from build123d import *

# Parameters (mm, degrees)
SKETCH_1_W             = 30
SKETCH_1_H             = 250
EXTRUDE_1_DEPTH        = 3
EXTRUDE_2_DEPTH        = 15
PATTERN_LINEAR_1_COUNT = 35
PATTERN_LINEAR_1_PITCH = 7


with BuildPart() as part:
    # 스케치1 → 보스-돌출1 (new body)
    with BuildSketch(Plane(origin=(0, 0, 0), x_dir=(1, 0, 0), z_dir=(0, 1, 0))):
        Rectangle(SKETCH_1_W, SKETCH_1_H)
    extrude(amount=EXTRUDE_1_DEPTH)

    # 스케치3 → 보스-돌출2 (add, symmetric)
    with BuildSketch(Plane(origin=(0, 0, 0), x_dir=(0, 0, -1), z_dir=(1, 0, 0))):
        Polygon((-125, 3), (-118, 6), (-118, 3), align=None)
    extrude_2 = extrude(amount=EXTRUDE_2_DEPTH, both=True)

    # 선형 패턴1: 보스-돌출2 ×35
    with Locations(*[(0, 0, -i * PATTERN_LINEAR_1_PITCH) for i in range(1, PATTERN_LINEAR_1_COUNT)]):
        add(extrude_2)


solid = part.part
Model file for the job. Use its own axes, mm. Give positions to 0.01 mm unless a question says otherwise; leave off trailing zeros. Order: outer loops, then holes, each group sorted by start corner. A loop starts at its lowest first (then second) coordinate and runs counter-clockwise, first axis right, second up. Notation, with made-up numbers: (-33, 38) - (-7, 38) arc R8 ccw to (-7, 47) - close; hole circle Ø2 at (53.25, -25). An arc over 180 degrees is marked (long way). Return JSON: item names as keys, results as strings.
1) Probe line 1 (Y direction, x = 1.5, z = -54.5); line 2 (Y direction, x = -9.5, z = 114). List the from-to ranges inside material, lowest first. Write a range as from..to.
Geometry says:
{"line 1": "0..4.93", "line 2": "0..4.71"}
2) Flat gauge pin, fed straight in: P1, Ø1.5, axis at x = 3.5, y = 4.5, coming from the -Z side. Where does the tip first touch, or does it go through?
Geometry says:
{"P1": "z = -120"}
3) Cut at C-C, the plane z = 38. Give the cut face in (x, y).
Geometry says:
{"outline": "(-15, 0) - (15, 0) - (15, 4.29) - (-15, 4.29) - close"}
4) Cut at A-A, the plane y = 4.5. Count the separate pieces of the cut face and the enclosed holes in it, plus the area to 4 significant figures.
Geometry says:
{"separate pieces": "35", "enclosed holes": "0", "area": "3,675 mm²"}
5) Pull direction Z, two halves, no side cores. Call faces 1 (the flat face through (0.2, 4.5, 121.5)), 2 (the flat face through (0.2, 4.5, 23.5)), 3 (the flat face through (0, 3, -123)): pulls with the +Z half, pulls with the -Z half, needs draft (parallel to the pull), parting line crosses it, or undercut.
Geometry says:
{"face 1": "pulls with the +Z half", "face 2": "undercut", "face 3": "needs draft"}
6) Cut at B-B, the plane z = 80.5. Give the cut face in (x, y).
Geometry says:
{"outline": "(-15, 0) - (15, 0) - (15, 4.07) - (-15, 4.07) - close"}
